Build history of the part. All positions in model axes, mm. A direction names the side the tool comes from. Round coordinates to 2 decimals unless told otherwise and drop trailing zeros. Order: outer loops, then holes, each group sorted by start corner. A loop starts at its lowest first (then second) coordinate and runs counter-clockwise, first axis right, second up. Notation, with made-up numbers: (80, 23) -> (105, 23) arc R9 ccw to (105, 39) -> close; hole circle Ø2 at (38.25, -4.5). An arc over 180 degrees is marked (long way). Use a Markdown table: item, result. Add a question column.
Item 1: Slice it at D-D, the plane z = 56.5. Give the cut face in (x, y).
Item 2: Slice it at C-C, the plane x = 7. Give the cut face in (y, z), plus the area to 3 significant figures.
Item 3: 3-axis set-ups, long thin cutter, end or side, ignore diameter. For faces 1 (the face through (-3, -150, -50.8)), 2 (the face through (166.79, -286.02, 28.36)), 3 (the face through (181.45, -160.43, 82.11)): which of +Z, -Z, +X, -X, +Y, -Y reach the whole face in a straight line?
Item 4: Pin check, flat tips, straight feed: pin 1 (11 mm diameter, centred on y = -158, z = -0.5, fed in from -X); pin 2 (1.5 mm diameter, centred on x = -167, y = -254, fed in from +Z); pin 3 (5 mm diameter, centred on x = 133, z = 37.5, fed in from +Y). Stop position of each tip, or through.
Item 5: Two-plate mould, pull along X, no slides. Class faces 4 (the face through (-209.817, -134.085, 0.806)), 5 (the face through (-190.5, -152, 0)), 6 (the face through (164, -266.7, -19)): released by +X, released by -X, zero draft, split by the parting line, or undercut.
Item 6: Slice it at B-B, the plane y = -216.5. Give the cut face in (x, z), plus the area to 3 significant figures.
Item 7: Probe L1, parallel to Z at x = -207, y = -152.4; L2, parallel to Z at x = -64.5, y = -103; L3, parallel to Y at x = -177, z = 5. List the from-to ranges inside material, lowest first.
Item 8: Slice it at A-A, the plane z = 0. Give the cut face in (x, y).
from build123d import *

# Parameters (mm, degrees)
F0_W     = 457.2
F0_H     = 101.6
F1_DEPTH = 304.8
F2_R     = 57.15
F3_DEPTH = 38.1
F4_R     = 7.133851
F4_R_2   = 11.398645
F5_DEPTH = 63.5
F6_DEPTH = 63.5
F7_R     = 18.332449
F8_DEPTH = 38.1


with BuildPart() as f1:
    # F0 (on Front) → F1 (new body)
    with BuildSketch(Plane.XZ):
        Rectangle(F0_W, F0_H)
    extrude(amount=F1_DEPTH)

    # F2 (on face) → F3 (cut)
    with BuildSketch(Plane.XZ.offset(304.8)):
        with Locations((-161.700301, -31.462707)):
            Circle(F2_R)
        with Locations((165.217001, -28.766797)):
            Circle(F2_R)
    extrude(amount=-F3_DEPTH, mode=Mode.SUBTRACT)

    # F4 (on face) → F5 (join)
    with BuildSketch(Plane.XY.offset(50.8)):
        with Locations((191.001311, -71.4375)):
            Circle(F4_R)
        with Locations((170.921057, -156.06603)):
            Circle(F4_R_2)
    extrude(amount=F5_DEPTH)

    # F4 (on face) → F6 (join)
    with BuildSketch(Plane.XY.offset(50.8)):
        with Locations((191.001311, -71.4375)):
            Circle(F4_R)
        with Locations((170.921057, -156.06603)):
            Circle(F4_R_2)
    extrude(amount=F6_DEPTH)

    # F7 (on face) → F8 (cut)
    with BuildSketch(Plane(origin=(-228.6, 0, 0), x_dir=(0, -1, 0), z_dir=(-1, 0, 0))):
        with Locations((152.4, 0)):
            Circle(F7_R)
    extrude(amount=-F8_DEPTH, mode=Mode.SUBTRACT)


solid = f1.part
Check sheet entries:
| question | item | result |
|---|---|---|
| 1 | outline | circle Ø22.8 at (170.92, -156.07); circle Ø14.27 at (191, -71.44) |
| 2 | outline | (-304.8, -50.8) -> (0, -50.8) -> (0, 50.8) -> (-304.8, 50.8) -> close |
| 2 | area | 31,000 mm2 |
| 3 | face 1 | -Z, +X, -X, +Y, -Y |
| 3 | face 2 | -Y |
| 3 | face 3 | +Z |
| 4 | pin 1 | x = -190.5 |
| 4 | pin 2 | z = 50.8 |
| 4 | pin 3 | y = 0 |
| 5 | face 4 | zero draft |
| 5 | face 5 | released by -X |
| 5 | face 6 | undercut |
| 6 | outline | (-228.6, -50.8) -> (228.6, -50.8) -> (228.6, 50.8) -> (-228.6, 50.8) -> close |
| 6 | area | 46,500 mm2 |
| 7 | L1 | -50.8 to -18.33, 18.33 to 50.8 |
| 7 | L2 | -50.8 to 50.8 |
| 7 | L3 | -266.7 to 0 |
| 8 | outline | (-228.6, -304.8) -> (-209.41, -304.8) -> (-209.41, -266.7) -> (-113.99, -266.7) -> (-113.99, -304.8) -> (115.83, -304.8) -> (115.83, -266.7) -> (214.6, -266.7) -> (214.6, -304.8) -> (228.6, -304.8) -> (228.6, 0) -> (-228.6, 0) -> (-228.6, -134.07) -> (-190.5, -134.07) -> (-190.5, -170.73) -> (-228.6, -170.73) -> close |
